Read the model definition and answer for the solid it produces. Units are mm, in the model's axes. Face numbers are marked on the shaded views. A direction names the side the tool comes from. Round coordinates to 2 decimals unless told otherwise and drop trailing zeros. Write each loop counter-clockwise with the first axis right and the second up, starting at its lowest first coordinate (ties: lowest second). Pieces come first, ordered by that corner, then holes. Notation, with made-up numbers: (77.25, 29.5) -> (125.25, 29.5) arc R29 cw to (125.25, 58.5) -> close; hole circle Ø10 at (86.5, 19.25). An arc over 180 degrees is marked (long way). Return JSON: item names as keys, results as strings. Group by question number.
(1) Straight lines are drawn through the part: line 1 (X direction, y = 9.75, z = 2.5); line 2 (X direction, y = 4, z = 5.75); line 3 (Y direction, x = -0.8, z = 11.5). For each, find the intervals that lie inside material, in ascending order.
(2) A cutting plane is placed at D-D on x = -1. Give the vertices of the cut face in (y, z).
(3) A cutting plane is placed at C-C on y = 0. Give the vertices of the cut face in (x, z).
(4) A cutting plane is placed at B-B on z = 14.25. Give the vertices of the cut face in (x, y).
(5) Given pin 1 (1.5 mm diameter, centred on y = 9.5, z = 4.5, fed in from +X); pin 2 (0.6 mm diameter, centred on y = 9, z = 5.5, fed in from -X); pin 3 (0.7 mm diameter, centred on y = 3, z = 8, fed in from +X), each flat-ended and moving along its own axis, determine where each tip first touches the part or whether it passes through.
(6) The mould has two halves that part along Y. Classify the marked faces 1, 2 and 3: released by +Y, released by -Y, zero draft, split by the parting line, or undercut.
(7) A cutting plane is placed at A-A on x = 1.8. Give the vertices of the cut face in (y, z).
(8) For the marked faces 4, 5 and 6, determine the directions among +Z, -Z, +X, -X, +Y, -Y from which every point of the face is accessible in a straight line to the end or side of a thin tool.
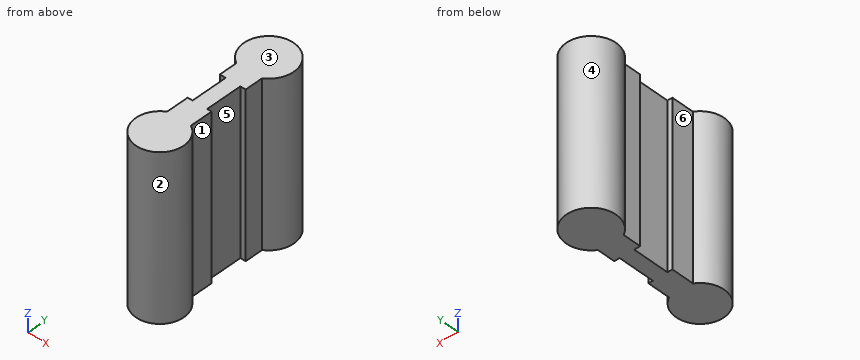
Autodesk Fusion 360 part; units mm, degrees
sketch "Sketch1" plane through (0, 0, 0) normal (0, 0, 1) x (1, 0, 0)
  circle A0 centre (0, 0) radius 2.5
  line L0 (-1.35, 2.1042) -> (-1.35, 10.1042)
  line L1 (1.35, 2.1042) -> (1.35, 10.1042)
  circle A1 centre (0, 12.3262) radius 2.6
  dimension "d1" = 5
  dimension "d4" = 1.35
  dimension "d5" = 5.2
  dimension "d6" = 8
  dimension "d7" = 8
  dimension "d12" = 2.7
extrude "Extrude1" add sketch "Sketch1" along normal blind 17
sketch "Sketch2" plane through (0, 0, 17) normal (0, 0, 1) x (-1, 0, 0)
  arc A0 (1.35, -2.1042) -> (-1.35, -2.1042) centre (0, 0) ccw
  line L0 (-1.35, -2.1042) -> (-1.35, -10.1042)
  arc A1 (-1.35, -10.1042) -> (1.35, -10.1042) centre (0, -12.3262) ccw
  line L1 (1.35, -10.1042) -> (1.35, -2.1042)
  line L2 (1.35, -8.2485) -> (-1.35, -8.2485)
  line L3 (-1.35, -8.2485) -> (-1.35, -4.4962)
  line L4 (-1.35, -4.4962) -> (1.35, -4.4962)
  line L5 (1.35, -4.4962) -> (1.35, -8.2485)
  line L6 (0.7348, -8.2485) -> (0.7348, -4.4962)
  line L7 (-0.7891, -8.2485) -> (-0.7891, -4.4962)
  arc A2 (1.35, -2.1042) -> (-1.35, -2.1042) centre (0, 0) ccw
  circle A3 centre (0, 0) radius 2.5
  line L8 (1.25, -4.4962) -> (1.25, -2.1651)
  line L9 (-1.25, -4.4962) -> (-1.25, -2.1651)
  line L10 (1.35, -2.1042) -> (1.35, -4.4962)
  line L11 (-1.35, -4.4962) -> (-1.35, -2.1042)
  dimension "d13" = 2.5
  dimension "d14" = 1.25
extrude "Extrude2" cut sketch "Sketch2" against normal blind 17 contours L1 L4 A3 L8 L10 | L1 L2 L4 L5 L6 | L0 L4 A3 L9 L11 | L0 L2 L3 L4 L7
Checks:
{
 "1": {"line 1": "x = -1.35 to 1.35", "line 2": "x = -1.25 to 1.25", "line 3": "y = -2.37 to 4.5, 8.25 to 14.8"},
 "2": {"outline": "(-2.29, 0) -> (4.5, 0) -> (4.5, 17) -> (-2.29, 17) -> close; (8.25, 0) -> (14.73, 0) -> (14.73, 17) -> (8.25, 17) -> close"},
 "3": {"outline": "(-2.5, 0) -> (2.5, 0) -> (2.5, 17) -> (-2.5, 17) -> close"},
 "4": {"outline": "(-1.35, 8.25) -> (-0.73, 8.25) -> (-0.73, 4.5) -> (-1.25, 4.5) -> (-1.25, 2.17) arc R2.5 ccw (long way) to (1.25, 2.17) -> (1.25, 4.5) -> (0.79, 4.5) -> (0.79, 8.25) -> (1.35, 8.25) -> (1.35, 10.1) arc R2.6 ccw (long way) to (-1.35, 10.1) -> close"},
 "5": {"pin 1": "stops at x = 1.57", "pin 2": "stops at x = -1.35", "pin 3": "stops at x = 1.25"},
 "6": {"face 1": "undercut", "face 2": "undercut", "face 3": "zero draft"},
 "7": {"outline": "(-1.73, 0) -> (1.73, 0) -> (1.73, 17) -> (-1.73, 17) -> close; (10.45, 0) -> (14.2, 0) -> (14.2, 17) -> (10.45, 17) -> close"},
 "8": {"face 4": "+Z, -Z", "face 5": "+Z, -Z, +X", "face 6": "+Z, -Z, -X"}
}
